Answer from the drawing. Dimensions are ordinates in mm from the lowest x, y and z of the part. Give positions to 0.01 mm unless a question says otherwise; leave off trailing zeros. Loops run counter-clockwise (first coordinate to the right, second up) from the corner with the lowest first, then second, coordinate; pieces in that order, holes last. Notation, with made-up numbers: M -31,72.5 L -22,72.5 A30 ccw -22,106.5 Z; hole C 84,52.25 d9. An arc over 180 degrees is marked long. Return JSON: item names as keys, results as strings. Group by question number.
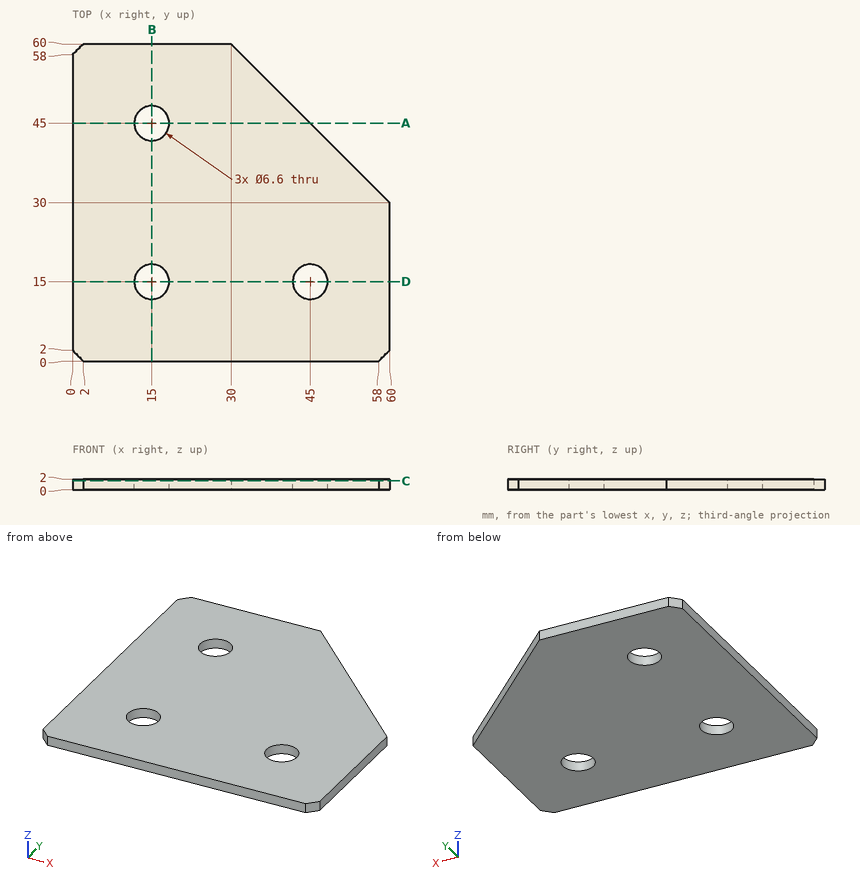
1. Find section B-B (x = 15). Write down the section's boundary in (y, z).
2. Straight lines are drawn through the part: line 1 along Y through (x, z) = (15, 0.55); line 2 along X through (y, z) = (18, 0.45). For each, find the intervals that lie inside material, in ascending order.
3. Find section C-C (z = 1.65). Write down the section's boundary in (x, y).
4. Flat-ended cylindrical pins translate along their axes: P1, Ø5.5, axis at x = 15, y = 45, coming from the +Z side; P2, Ø1, axis at x = 45.5, z = 1.5, coming from the +Y side. Find the tip coordinate at first contact, or state that the pin passes through.
5. Find section A-A (y = 45). Write down the section's boundary in (x, z), and give its area (3 significant figures).
Result:
{
 "1": {"outline": "M 0,0 L 11.7,0 L 11.7,2 L 0,2 Z; M 18.3,0 L 41.7,0 L 41.7,2 L 18.3,2 Z; M 48.3,0 L 60,0 L 60,2 L 48.3,2 Z"},
 "2": {"line 1": "y = 0 to 11.7, 18.3 to 41.7, 48.3 to 60", "line 2": "x = 0 to 13.63, 16.37 to 43.63, 46.37 to 60"},
 "3": {"outline": "M 0,2 L 2,0 L 58,0 L 60,2 L 60,30 L 30,60 L 2,60 L 0,58 Z; hole C 15,15 d6.6; hole C 15,45 d6.6; hole C 45,15 d6.6"},
 "4": {"P1": "passes through", "P2": "stops at y = 45"},
 "5": {"outline": "M 0,0 L 11.7,0 L 11.7,2 L 0,2 Z; M 18.3,0 L 45,0 L 45,2 L 18.3,2 Z", "area": "76.8 mm2"}
}
